from build123d import *

# Parameters (mm, degrees)
BOSS_EXTRUDE1_DEPTH            = 12
CUT_EXTRUDE1_DEPTH             = 34
F_3_6_3_6_DIAMETER_HOLE1_D     = 3.6
F_3_6_3_6_DIAMETER_HOLE1_DEPTH = 10
F_3_6_3_6_DIAMETER_HOLE1_TIP   = 1.081549114


with BuildPart() as part:
    # Sketch1 → Boss-Extrude1 (new body)
    with BuildSketch(Plane(origin=(0, 0, 0), x_dir=(1, 0, 0), z_dir=(0, 1, 0))):
        with BuildLine():
            Line((-36, 31), (36, 31))
            ThreePointArc((36, 31), (39.535533906, 29.535533906), (41, 26))
            Line((41, 26), (41, -26))
            ThreePointArc((41, -26), (39.535533906, -29.535533906), (36, -31))
            Line((36, -31), (-36, -31))
            ThreePointArc((-36, -31), (-39.535533906, -29.535533906), (-41, -26))
            Line((-41, -26), (-41, 26))
            ThreePointArc((-41, 26), (-39.535533906, 29.535533906), (-36, 31))
        make_face()
    extrude(amount=BOSS_EXTRUDE1_DEPTH)

    # Sketch2 → Cut-Extrude1 (cut, symmetric)
    with BuildSketch(Plane(origin=(0, 0, 0), x_dir=(0, 0, -1), z_dir=(1, 0, 0))):
        with BuildLine():
            Line((-10.197159549, 8), (-8.802840451, 8))
            ThreePointArc((-8.802840451, 8), (0, 1.7), (8.802840451, 8))
            Line((8.802840451, 8), (10.197159549, 8))
            ThreePointArc((10.197159549, 8), (20.520457794, 1.825131712), (28.3, 11))
            Line((28.3, 11), (28.3, 17.866390663))
            Line((28.3, 17.866390663), (-28.3, 17.866390663))
            Line((-28.3, 17.866390663), (-28.3, 11))
            ThreePointArc((-28.3, 11), (-20.520457794, 1.825131712), (-10.197159549, 8))
        make_face()
    extrude(amount=CUT_EXTRUDE1_DEPTH, both=True, mode=Mode.SUBTRACT)

    # Ø3.6 (3.6) Diameter Hole1
    with Locations(Plane(origin=(0, 12, 0), x_dir=(1, 0, 0), z_dir=(0, 1, 0))):
        with Locations((-37.5, 25), (-37.5, -25), (37.5, -25), (37.5, 25)):
            Hole(F_3_6_3_6_DIAMETER_HOLE1_D / 2, depth=F_3_6_3_6_DIAMETER_HOLE1_DEPTH)
            with Locations((0, 0, -(F_3_6_3_6_DIAMETER_HOLE1_DEPTH + F_3_6_3_6_DIAMETER_HOLE1_TIP / 2))):  # 118° drill point
                Cone(0, F_3_6_3_6_DIAMETER_HOLE1_D / 2, F_3_6_3_6_DIAMETER_HOLE1_TIP, mode=Mode.SUBTRACT)


solid = part.part
Here's how the part is built. I have some questions about the finished solid (model axes, mm). A direction names the side the tool comes from. Coordinates: 2 decimals unless noted, no trailing zeros. Write each loop counter-clockwise with the first axis right and the second up, starting at its lowest first coordinate (ties: lowest second). Pieces come first, ordered by that corner, then holes.
1) If we section it at B-B (y = 3.5): List the corners of the cut face in (x, z) for me.
Filled in:
outline: (-41, -26) arc R5 ccw to (-36, -31) - (36, -31) arc R5 ccw to (41, -26) - (41, 26) arc R5 ccw to (36, 31) - (-36, 31) arc R5 ccw to (-41, 26) - close; hole circle Ø3.6 at (-37.5, -25); hole circle Ø3.6 at (-37.5, 25); hole (-34, -24.5) - (34, -24.5) - (34, -13.5) - (-34, -13.5) - close; hole (-34, -5.5) - (34, -5.5) - (34, 5.5) - (-34, 5.5) - close; hole (-34, 13.5) - (34, 13.5) - (34, 24.5) - (-34, 24.5) - close; hole circle Ø3.6 at (37.5, -25); hole circle Ø3.6 at (37.5, 25)
2) Thinking about a two-plate mould opening in Z: for faces 3 (the face through (1, 6, 31)), 4 (the face through (-37.73, 1.106, -25.211)), 5 (the face through (-40, 6, -29)), which applies, +Z half, -Z half, draft (parallel to the pull), parting line (faces both ways), or undercut?
Filled in:
face 3: +Z half
face 4: undercut
face 5: -Z half
3) I'm going to push flat-ended pins straight in: pin 1 (10 mm diameter, centred on x = 12, z = 21.5, fed in from +Y); pin 2 (4 mm diameter, centred on x = -37.5, z = 25, fed in from -Y); pin 3 (3 mm diameter, centred on x = 37.5, z = 25, fed in from +Y); pin 4 (12 mm diameter, centred on x = 1.5, z = 19.5, fed in from +Y). Where does each tip first touch, or does it pass through?
Filled in:
pin 1: stops at y = 5.5
pin 2: stops at y = 0
pin 3: stops at y = 1.82
pin 4: stops at y = 4.35
4) If I drill on line 1 (X direction, y = 7.25, z = 25); line 2 (Z direction, x = -37.5, y = 5.75); line 3 (Z direction, x = 18, y = 3), over which ranges is the centre line in solid material (lowest first)?
Filled in:
line 1: x = -41 to -39.3, -35.7 to -34, 34 to 35.7, 39.3 to 41
line 2: z = -30.77 to -26.8, -23.2 to 23.2, 26.8 to 30.77
line 3: z = -31 to -23.74, -14.26 to -4.74, 4.74 to 14.26, 23.74 to 31
5) Which directions (+Z, -Z, +X, -X, +Y, -Y) give clear straight access to the entire face, cutting with the end or side of a thin tool? Please do faces 1 (the face through (-1, 6, -31)), 2 (the face through (-38.468, 6.93, -26.518)).
Filled in:
face 1: -Z, +X, -X, +Y, -Y
face 2: +Y
6) If we section it at A-A (x = -7): List the corners of the cut face in (y, z) for me, plus the area to 3 significant figures.
Filled in:
outline: (0, -31) - (12, -31) - (12, -28.3) - (11, -28.3) arc R9.3 cw to (8, -10.2) - (8, -8.8) arc R9.3 cw to (8, 8.8) - (8, 10.2) arc R9.3 cw to (11, 28.3) - (12, 28.3) - (12, 31) - (0, 31) - close
area: 275 mm2
